Can you work these out from the model? Positions are in its coordinate system, mm. Face numbers are marked on the shaded views. A direction names the side the tool comes from. Coordinates: 2 decimals unless noted, no trailing zeros. Write each loop counter-clockwise with the first axis right and the second up, starting at its lowest first coordinate (ties: lowest second). Pieces come first, ordered by that corner, then holes. Notation, with made-up numbers: (28, -36) -> (53, -36) arc R20 ccw to (53, -31) -> close; hole circle Ø8 at (-32.5, 15.25). An arc over 180 degrees is marked (long way). Answer as CSV lines item,"result". Start each with the question number.
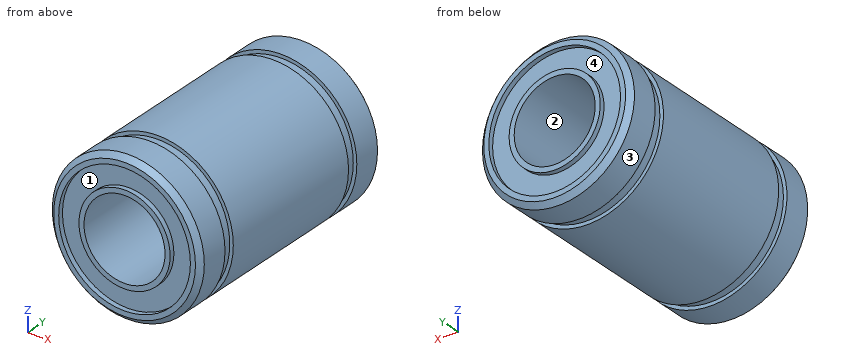
```python
from build123d import *

# Parameters (mm, degrees)
SKETCH2_R          = 6.5
SKETCH2_R_2        = 4.5
CUT_EXTRUDE1_DEPTH = 0.5


with BuildPart() as part:
    # Sketch1 → Body (revolve)
    with BuildSketch(Plane.XY):
        Polygon((4, -12), (4, 12), (7, 12), (7.5, 11.5), (7.5, 8.75), (7.15, 8.75), (7.15, 7.65), (7.5, 7.65), (7.5, -7.65), (7.15, -7.65), (7.15, -8.75), (7.5, -8.75), (7.5, -11.5), (7, -12), align=None)
    revolve(axis=Axis((0, 12, 0), (0, -1, 0)))

    # Sketch2 → Cut-Extrude1 (cut)
    with BuildSketch(Plane(origin=(0, 12, 0), x_dir=(1, 0, 0), z_dir=(0, 1, 0))):
        Circle(SKETCH2_R)
        Circle(SKETCH2_R_2, mode=Mode.SUBTRACT)
    cut_extrude1 = extrude(amount=-CUT_EXTRUDE1_DEPTH, mode=Mode.SUBTRACT)

    # Mirror1: Cut-Extrude1 across plane
    add(cut_extrude1.mirror(Plane.ZX), mode=Mode.SUBTRACT)


solid = part.part
```
Q1. Which directions (+Z, -Z, +X, -X, +Y, -Y) give clear straight access to the entire face, cutting with the end or side of a thin tool? Please do the marked faces 1 and 2.
Q2. For pin 1 (4 mm diameter, centred on x = -2, z = 2.5, fed in from +Y); pin 2 (1 mm diameter, centred on y = 7.5, z = -1, fed in from -X); pin 3 (1.5 mm diameter, centred on x = 4.5, z = -3, fed in from -Y); pin 4 (3 mm diameter, centred on x = -3, y = -7, fed in from -Z), each with a flat end and sliding along its axis, tell me the tip position at first contact or that it passes through.
Q3. Imagine slicing it at B-B (y = 10). Write out the boundary of the cut face in (x, z).
Q4. If we mould it in two halves opening along Z, with no side actions, what happens to the marked faces 3 and 4? For each: released by +Z, released by -Z, zero draft, split by the parting line, or undercut.
Q5. I need wall thicknesses on L1, parallel to Z at x = 0, y = -11.85; L2, parallel to Z at x = 0, y = -11.75; L3, parallel to Z at x = 0, y = 5.75. Which ranges of each line are inside material? Lowest first, please.
Q6. Imagine slicing it at A-A (y = -8). Write out the boundary of the cut face in (x, z).
Entries:
1,face 1,"-Y"
1,face 2,"+Y, -Y"
2,pin 1,"y = 12"
2,pin 2,"x = -7.48"
2,pin 3,"y = -11.5"
2,pin 4,"z = -7.35"
3,outline,"circle Ø15 at (0, 0); hole circle Ø8 at (0, 0)"
4,face 3,"split by the parting line"
4,face 4,"undercut"
5,L1,"-7.15 to -6.5, -4.5 to -4, 4 to 4.5, 6.5 to 7.15"
5,L2,"-7.25 to -6.5, -4.5 to -4, 4 to 4.5, 6.5 to 7.25"
5,L3,"-7.5 to -4, 4 to 7.5"
6,outline,"circle Ø14.3 at (0, 0); hole circle Ø8 at (0, 0)"
